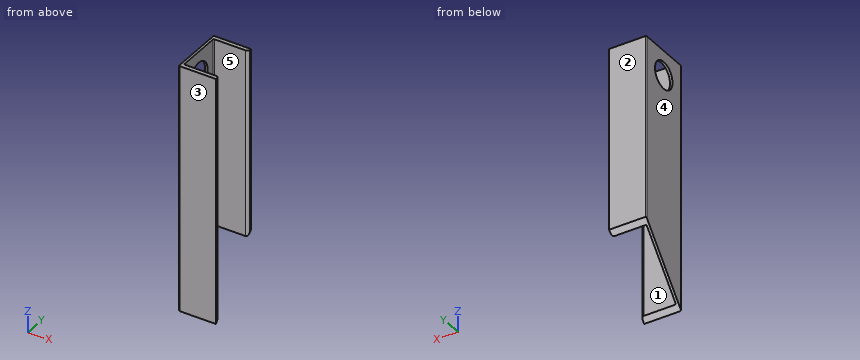
```python
from build123d import *

# Parameters (mm, degrees)
BOSS_EXTRUDE1_DEPTH = 300
CUT_EXTRUDE1_REACH  = 307.146
FILLET1_R           = 3
FILLET2_R           = 1
SKETCH4_R           = 16.5
CUT_EXTRUDE2_DEPTH  = 10


with BuildPart() as part:
    # Sketch1 → Boss-Extrude1 (new body)
    with BuildSketch(Plane.XY):
        Polygon((0, 33), (0, -33), (45, -33), (45, -27.9), (3, -27.9), (3, 27.9), (45, 27.9), (45, 33), align=None)
    extrude(amount=BOSS_EXTRUDE1_DEPTH)

    # Sketch3 → Cut-Extrude1 (cut, up to next)
    with BuildSketch(Plane.ZY, mode=Mode.PRIVATE) as cut_extrude1_sk1:
        Polygon((0, -33), (0, 33), (78.655737111, 33), align=None)
    cut_extrude1_tool1 = extrude(cut_extrude1_sk1.sketch, amount=-CUT_EXTRUDE1_REACH, mode=Mode.PRIVATE) & part.part
    add(cut_extrude1_tool1.solids().sort_by_distance((0, 11, 26.218579))[0], mode=Mode.SUBTRACT)

    # Fillet1
    fillet1_edges = [part.edges().sort_by_distance(p)[0] for p in [
        (45, -27.9, 153.038971661),
        (45, 27.9, 186.288896894),
    ]]
    fillet(fillet1_edges, radius=FILLET1_R)

    # Fillet2
    fillet2_edges = [part.edges().sort_by_distance(p)[0] for p in [
        (3, -27.9, 153.038971661),
        (0, -33, 150),
        (0, 33, 189.327868556),
        (3, 27.9, 186.288896894),
    ]]
    fillet(fillet2_edges, radius=FILLET2_R)

    # Sketch4 → Cut-Extrude2 (cut)
    with BuildSketch(Plane.ZY):
        with Locations(Location((270, 0, 0), (0, 0, 270))):
            Circle(SKETCH4_R)
    extrude(amount=-CUT_EXTRUDE2_DEPTH, mode=Mode.SUBTRACT)


solid = part.part
```
The model under review builds one solid part; all positions refer to its coordinate system, in mm. Face numbers are marked on the shaded views. A direction names the side the tool comes from. Coordinates: 2 decimals unless noted, no trailing zeros. Write each loop counter-clockwise with the first axis right and the second up, starting at its lowest first coordinate (ties: lowest second). Pieces come first, ordered by that corner, then holes.
1) Clearance check with a flat-ended pin moving along its axis: pin 1 Ø5 at (y, z) = (5, 254.5) entering from +X. State where the tip first meets the part, or that it passes through.
2) We need section B-B on y = -12. State the section outline as (x, z) points, then the cut area to 3 significant figures.
3) We need section A-A on z = 270. State the section outline as (x, y) points, then the cut area to 3 significant figures.
4) To check wall thickness, follow probe 1 along Y at (x, z) = (24, 196.5); probe 2 along X at (y, z) = (-24.5, 241); probe 3 along Y at (x, z) = (13.5, 12). State the ranges of each line that lie inside material, in increasing order.
5) We need section C-C on x = 36. State the section outline as (y, z) points, then the cut area to 3 significant figures.
6) Machinability: for the marked faces 4 and 5, which of the approach directions +Z, -Z, +X, -X, +Y, -Y give a long, thin tool a straight path to every point of the face, cutting with its end or side? Answer none if there is none.
7) The part is to be moulded in two halves that separate along Y. For the marked faces 1, 2 and 3, say which applies: pulls with the +Y half, pulls with the -Y half, needs draft (parallel to the pull), parting line crosses it, or undercut.
8) We need section D-D on z = 32. State the section outline as (x, y) points, then the cut area to 3 significant figures.
Answer list:
1. pin 1: stops at x = 3
2. outline: (0, 25.03) - (3, 25.03) - (3, 258.68) - (0, 258.68) - close; (0, 281.32) - (3, 281.32) - (3, 300) - (0, 300) - close
2. area: 757 mm2
3. outline: (0, -32) arc R1 ccw to (1, -33) - (45, -33) - (45, -30.9) arc R3 ccw to (42, -27.9) - (4, -27.9) arc R1 cw to (3, -26.9) - (3, -16.5) - (0, -16.5) - close; (0, 16.5) - (3, 16.5) - (3, 26.9) arc R1 cw to (4, 27.9) - (42, 27.9) arc R3 ccw to (45, 30.9) - (45, 33) - (1, 33) arc R1 ccw to (0, 32) - close
3. area: 524 mm2
4. probe 1: y = -33 to -27.9, 27.9 to 33
4. probe 2: x = 0 to 3
4. probe 3: y = -33 to -27.9
5. outline: (-33, 0) - (-27.9, 6.08) - (-27.9, 300) - (-33, 300) - close; (27.9, 72.58) - (33, 78.66) - (33, 300) - (27.9, 300) - close
5. area: 2,660 mm2
6. face 4: +Z, -Z, -X, +Y, -Y
6. face 5: +Z, -Z, +X
7. face 1: undercut
7. face 2: pulls with the +Y half
7. face 3: pulls with the -Y half
8. outline: (0, -32) arc R1 ccw to (1, -33) - (45, -33) - (45, -30.9) arc R3 ccw to (42, -27.9) - (4, -27.9) arc R1 cw to (3, -26.9) - (3, -6.15) - (0, -6.15) - close
8. area: 293 mm2
